from build123d import *

# Parameters (mm, degrees)
BOSS_EXTRUDE1_DEPTH      = 14
BOSS_EXTRUDE2_DEPTH      = 7
BOSS_EXTRUDE2_DEPTH_BACK = 7
SKETCH3_R                = 14.5
BOSS_EXTRUDE3_DEPTH      = 24.9
BOSS_EXTRUDE3_DEPTH_BACK = 24.9


with BuildPart() as part:
    # Sketch1 → Boss-Extrude1 (new body)
    with BuildSketch(Plane(origin=(0, 0, 0), x_dir=(1, 0, 0), z_dir=(0, 1, 0))):
        with BuildLine():
            Line((-33, -30), (33, -30))
            ThreePointArc((33, -30), (40.071067812, -27.071067812), (43, -20))
            Line((43, -20), (43, 20))
            ThreePointArc((43, 20), (40.071067812, 27.071067812), (33, 30))
            Line((33, 30), (-33, 30))
            ThreePointArc((-33, 30), (-40.071067812, 27.071067812), (-43, 20))
            Line((-43, 20), (-43, -20))
            ThreePointArc((-43, -20), (-40.071067812, -27.071067812), (-33, -30))
        make_face()
    extrude(amount=BOSS_EXTRUDE1_DEPTH)

    # Sketch2 → Boss-Extrude2 (add, two sides)
    with BuildSketch(Plane(origin=(0, 0, 0), x_dir=(0, 0, -1), z_dir=(1, 0, 0))) as boss_extrude2_sk:
        Polygon((-41.005924481, 59.247123846), (-28.881994187, 14), (18.033320997, 14), (-14.442631645, 70.25), align=None)
    extrude(amount=BOSS_EXTRUDE2_DEPTH)
    extrude(boss_extrude2_sk.sketch, amount=-BOSS_EXTRUDE2_DEPTH_BACK)

    # Sketch3 → Boss-Extrude3 (add, two sides)
    with BuildSketch(Plane(origin=(0, 0, 0), x_dir=(0, 0, -1), z_dir=(1, 0, 0))) as boss_extrude3_sk:
        with Locations((-27, 63)):
            Circle(SKETCH3_R)
    extrude(amount=BOSS_EXTRUDE3_DEPTH)
    extrude(boss_extrude3_sk.sketch, amount=-BOSS_EXTRUDE3_DEPTH_BACK)

    # Sketch4 → Cut-Revolve1 (revolve, cut)
    with BuildSketch(Plane.XY.offset(20)):
        Polygon((-33, 0), (-38.5, 0), (-38.5, 12.7), (-42, 12.7), (-42, 14), (-33, 14), align=None)
    revolve(axis=Axis((-33, 14, 20), (0, -1, 0)), mode=Mode.SUBTRACT)

    # Sketch5 → Cut-Revolve2 (revolve, cut)
    with BuildSketch(Plane.XY.offset(-20)):
        Polygon((-33, 0), (-38.5, 0), (-38.5, 12.7), (-42, 12.7), (-42, 14), (-33, 14), align=None)
    revolve(axis=Axis((-33, 14, -20), (0, -1, 0)), mode=Mode.SUBTRACT)

    # Sketch6 → Cut-Revolve3 (revolve, cut)
    with BuildSketch(Plane.XY.offset(20)):
        Polygon((33, 0), (27.5, 0), (27.5, 12.7), (24, 12.7), (24, 14), (33, 14), align=None)
    revolve(axis=Axis((33, 14, 20), (0, -1, 0)), mode=Mode.SUBTRACT)

    # Sketch7 → Cut-Revolve4 (revolve, cut)
    with BuildSketch(Plane.XY.offset(-20)):
        Polygon((33, 0), (27.5, 0), (27.5, 12.7), (24, 12.7), (24, 14), (33, 14), align=None)
    revolve(axis=Axis((33, 14, -20), (0, -1, 0)), mode=Mode.SUBTRACT)

    # Sketch8 → Cut-Revolve5 (revolve, cut)
    with BuildSketch(Plane.XY.offset(27)):
        Polygon((-24.9, 63), (-24.9, 74.5), (-24.611324865, 74), (24.611324865, 74), (24.9, 74.5), (24.9, 63), align=None)
    revolve(axis=Axis((24.9, 63, 27), (-1, 0, 0)), mode=Mode.SUBTRACT)

    # Sketch9 → Revolve1 (revolve)
    with BuildSketch(Plane.XY.offset(27)):
        Polygon((-24.9, 71.3), (-24.6, 71), (24.6, 71), (24.9, 71.3), (24.9, 73.7), (24.6, 74), (-24.6, 74), (-24.9, 73.7), align=None)
    revolve(axis=Axis((24.9, 63, 27), (-1, 0, 0)))


solid = part.part
The model under review builds one solid part; all positions refer to its coordinate system, in mm. A direction names the side the tool comes from. Give positions to 0.01 mm unless a question says otherwise; leave off trailing zeros. Write each loop counter-clockwise with the first axis right and the second up, starting at its lowest first coordinate (ties: lowest second). Pieces come first, ordered by that corner, then holes.
1. For P1, Ø14.5, axis at x = -33, z = 20, coming from the -Y side; P2, Ø10, axis at x = 33, z = 20, coming from the +Y side; P3, Ø3, axis at x = 29.5, z = -17.5, coming from the +Y side; P4, Ø1, axis at x = -30, z = -4.5, coming from the +Y side, all flat-tipped, find the tip position at first contact; note any pin that passes through.
2. Add section A-A, the plane x = -16. Write out the cut boundary in (y, z).
3. Tool access review of faces 3 (the flat face through (24.9, 60, 35)), 4 (the flat face through (0, 7, 30)), 5 (the cylindrical face through (39.633, 13.359, -26.083)), 6 (the cylindrical face through (-27.505, 6.439, 19.758)): name each direction out of +Z, -Z, +X, -X, +Y, -Y from which nothing blocks a thin tool from reaching the whole face with its end or side.
4. Wall thickness on L1, parallel to X at y = 13.15, z = 20; L2, parallel to Z at x = -33, y = 8.75; L3, parallel to Z at x = -34, y = 10: over which ranges is each line inside the solid? List them lowest first.
5. Add section B-B, the plane y = 9.5. Write out the cut boundary in (x, z), plus the area to 3 significant figures.
6. Draft analysis for pull direction Y (two halves, no side actions). For faces 1 (the cylindrical face through (39.99, 6.9, 27.15)), 2 (the flat face through (-10, 14, 0)), state which applies: +Y half, -Y half, draft (parallel to the pull), parting line (faces both ways), or undercut.
7. Add section C-C, the plane z = 7. Write out the cut boundary in (x, y).
Worked answers:
1. P1: stops at y = 0
1. P2: passes through
1. P3: stops at y = 12.7
1. P4: stops at y = 14
2. outline: (0, -30) - (14, -30) - (14, 30) - (0, 30) - close; circle Ø29 at (63, 27); hole circle Ø16 at (63, 27)
3. face 3: +Z, -Z, +X, +Y
3. face 4: +Z, +X, -X, -Y
3. face 5: +Y
3. face 6: +Y, -Y
4. L1: x = -43 to -42, -24 to 24, 42 to 43
4. L2: z = -30 to -25.5, -14.5 to 14.5, 25.5 to 30
4. L3: z = -29.95 to -25.41, -14.59 to 14.59, 25.41 to 29.95
5. outline: (-43, -20) arc R10 ccw to (-33, -30) - (33, -30) arc R10 ccw to (43, -20) - (43, 20) arc R10 ccw to (33, 30) - (-33, 30) arc R10 ccw to (-43, 20) - close; hole circle Ø11 at (-33, -20); hole circle Ø11 at (-33, 20); hole circle Ø11 at (33, -20); hole circle Ø11 at (33, 20)
5. area: 4,690 mm2
6. face 1: draft
6. face 2: undercut
7. outline: (-43, 0) - (43, 0) - (43, 14) - (7, 14) - (7, 57.36) - (-7, 57.36) - (-7, 14) - (-43, 14) - close
